Input: part model. Units: mm. Frame: model coordinates. A direction names the side the tool comes from. Give positions to 0.01 mm unless a question says otherwise; leave off trailing zeros. Write each loop counter-clockwise with the first axis right and the second up, starting at its lowest first coordinate (ties: lowest second). Pieces come first, ordered by that corner, then holes. Notation, with made-up numbers: (-4.5, -35.75) -> (24.5, -35.75) arc R19 ccw to (24.5, -19.75) -> close; hole circle Ø10 at (2, -38). An arc over 180 degrees is marked (long way). Return JSON: item names as keys, results as strings. Group by question number.
Item 1: Set-up query: faces 4 (the face through (7.55, -1.39, 0.99)), 5 (the face through (5, -4.5, 1)), 6 (the face through (2.675, 5, 1)). Return all of +Z, -Z, +X, -X, +Y, -Y with unobstructed straight access to the full face (end or side cutting, diameter ignored); none if empty.
Item 2: Section A-A, the plane x = 5.25. Return loops of the section in (y, z).
Item 3: Pin query (flat end, axial travel): P1, Ø1, axis at x = 4.5, z = 0.5, coming from the +Y side; P2, Ø0.5, axis at y = -5, z = 1, coming from the +X side; P3, Ø1, axis at x = 5.5, z = 1, coming from the -Y side. Return the tip coordinate at first contact, or that it passes through.
Item 4: Section B-B, the plane z = 0.2. Return loops of the section in (x, y).
Item 5: Section D-D, the plane x = 9. Return loops of the section in (y, z), then the cut area to 3 significant figures.
Item 6: Line query: line 1 (Y direction, x = 4, z = 0.3); line 2 (Y direction, x = 3, z = 0.4); line 3 (X direction, y = 2, z = 1). Output: solid intervals per line, ascending. Write a range as [from, to].
Item 7: Mould query, pull axis Y, two halves, no side actions, for faces 1 (the face through (7.568, 1.356, 0.986)), 2 (the face through (0.76, 4.07, 0.99)), 3 (the face through (10.08, -4.26, 1.01)). Classes: released by +Y, released by -Y, zero draft, split by the parting line, or undercut.
Item 8: Section C-C, the plane y = 2.5. Return loops of the section in (x, z).
from build123d import *

# Parameters (mm, degrees)
BOSS_EXTRU_1_DEPTH = 2
CONG_1_R           = 4
CONG_2_R           = 1


with BuildPart() as part:
    # Esquisse1 → Boss.-Extru.1 (new body)
    with BuildSketch(Plane.XY):
        Polygon((0, 5.5), (2.675426481, 5.5), (2.675426481, 4.5), (7.775426481, 4.5), (7.775426481, 4.7), (10.350852961, 4.5), (10.350852961, -4.5), (7.775426481, -4.7), (7.775426481, -4.5), (2.675426481, -4.5), (2.675426481, -5.5), (0, -5.5), align=None)
        Polygon((2, 0), (3.58771324, -2.75), (6.763139721, -2.75), (8.350852961, 0), (6.763139721, 2.75), (3.58771324, 2.75), align=None, mode=Mode.SUBTRACT)
    extrude(amount=BOSS_EXTRU_1_DEPTH)

    # Congé1
    # the kernel refuses this fillet: 4 mm, written as the material it takes off along each edge
    with BuildSketch(Plane(origin=(0, -5.5, -9.435804481), x_dir=(1, 0, 0), z_dir=(0, 0, 1))) as cong_1_piece_1:
        with BuildLine():
            CenterArc((4, 3.774321792), CONG_1_R, 180, 70.661811314)
            Line((0, 3.774321792), (-0.08, 3.774321792))
            Line((-0.08, 3.774321792), (-0.08, 0))
            Line((-0.08, 0), (0, -0.08))
            ThreePointArc((0, -0.08), (1.33771324, -0.08), (2.64893501, -0.075486436))
            Line((2.64893501, -0.075486436), (2.675426481, 0))
        make_face()
    extrude(amount=20.871608961, mode=Mode.SUBTRACT)
    with BuildSketch(Plane(origin=(0, 5.5, -9.435804481), x_dir=(1, 0, 0), z_dir=(0, 0, 1))) as cong_1_piece_2:
        with BuildLine():
            CenterArc((4, -3.774321792), CONG_1_R, 109.338188686, 70.661811314)
            Line((0, -3.774321792), (-0.08, -3.774321792))
            Line((-0.08, -3.774321792), (-0.08, 0))
            Line((-0.08, 0), (0, 0.08))
            ThreePointArc((0, 0.08), (1.33771324, 0.08), (2.64893501, 0.075486436))
            Line((2.64893501, 0.075486436), (2.675426481, 0))
        make_face()
    extrude(amount=20.871608961, mode=Mode.SUBTRACT)

    # Congé2
    cong_2_edges = [part.edges().sort_by_distance(p)[0] for p in [
        (10.350852961, 4.5, 1),
        (10.350852961, -4.5, 1),
    ]]
    fillet(cong_2_edges, radius=CONG_2_R)


solid = part.part
Answer below:
{
 "1": {"face 4": "+Z, -Z", "face 5": "+Z, -Z, -Y", "face 6": "+Z, -Z, +Y"},
 "2": {"outline": "(-4.5, 0) -> (-2.75, 0) -> (-2.75, 2) -> (-4.5, 2) -> close; (2.75, 0) -> (4.5, 0) -> (4.5, 2) -> (2.75, 2) -> close"},
 "3": {"P1": "stops at y = 4.5", "P2": "stops at x = 2.68", "P3": "stops at y = -4.5"},
 "4": {"outline": "(0, -1.73) arc R4 ccw to (2.68, -5.5) -> (2.68, -4.5) -> (7.78, -4.5) -> (7.78, -4.7) -> (9.43, -4.57) arc R1 ccw to (10.35, -3.57) -> (10.35, 3.57) arc R1 ccw to (9.43, 4.57) -> (7.78, 4.7) -> (7.78, 4.5) -> (2.68, 4.5) -> (2.68, 5.5) arc R4 ccw to (0, 1.73) -> close; hole (2, 0) -> (3.59, -2.75) -> (6.76, -2.75) -> (8.35, 0) -> (6.76, 2.75) -> (3.59, 2.75) -> close"},
 "5": {"outline": "(-4.6, 0) -> (4.6, 0) -> (4.6, 2) -> (-4.6, 2) -> close", "area": "18.4 mm2"},
 "6": {"line 1": "y = [-4.5, -2.75], [2.75, 4.5]", "line 2": "y = [-4.5, -1.73], [1.73, 4.5]", "line 3": "x = [0.01, 3.15], [7.2, 10.35]"},
 "7": {"face 1": "undercut", "face 2": "released by +Y", "face 3": "released by -Y"},
 "8": {"outline": "(0.08, 0) -> (3.44, 0) -> (3.44, 2) -> (0.08, 2) -> close; (6.91, 0) -> (10.35, 0) -> (10.35, 2) -> (6.91, 2) -> close"}
}
